Build history of the part. All positions in model axes, mm. Face numbers are marked on the shaded views. A direction names the side the tool comes from. Give positions to 0.01 mm unless a question says otherwise; leave off trailing zeros. Loops run counter-clockwise (first coordinate to the right, second up) from the corner with the lowest first, then second, coordinate; pieces in that order, holes last. Notation, with made-up numbers: (5, 35) -> (17, 35) arc R26 cw to (17, 69) -> close; hole circle Ø5 at (18, 71.5). An arc over 180 degrees is marked (long way). One line per question, with ' | ' between items. Start each with the question number.
(1) 3-axis set-ups, long thin cutter, end or side, ignore diameter. For the marked faces 1, 2 and 3: which of +Z, -Z, +X, -X, +Y, -Y reach the whole face in a straight line?
(2) Slice it at C-C, the plane y = 17. Write the cut outline in (x, z) (3 decimals), then the cut area to 3 significant figures.
(3) Slice it at A-A, the plane z = -3.5. Write the cut outline in (x, y) (3 decimals), then the cut area to 3 significant figures.
(4) Drill centre lines: L1, parallel to Y at x = -22.5, z = 29; L2, parallel to X at y = -26.5, z = -1.5 (3 decimals); L3, parallel to Y at x = 32.5, z = 24.5. Where is each one in solid material? Low to high. Write a range as from..to.
(5) Flat gauge pins, fed straight in: pin 1 Ø2 at (x, y) = (62, 24.5) entering from -Z; pin 2 Ø2 at (x, y) = (60.5, -25) entering from +Z (3 decimals); pin 3 Ø21 at (x, z) = (47.5, 46) entering from -Y; pin 4 Ø24.5 at (x, z) = (-1.5, 40) entering from -Y. Where does each tip first touch, or does it go through?
(6) Slice it at B-B, the plane y = -49.5. Write the cut outline in (x, z) (3 decimals), then the cut area to 3 significant figures.
```python
from build123d import *

# Parameters (mm, degrees)
F1_DEPTH = 63.5
F2_DEPTH = 25.4
F3_DEPTH = 7.9375
F5_R     = 6.35


with BuildPart() as f1:
    # F0 (on Front) → F1 (new body, symmetric)
    with BuildSketch(Plane.XZ):
        Polygon((-41.275, -9.525), (41.275, -9.525), (41.275, 9.525), (22.225, 9.525), (-41.275, 9.525), align=None)
    extrude(amount=F1_DEPTH, both=True)

    # F0 (on Front) → F2 (join, symmetric)
    with BuildSketch(Plane.XZ):
        with BuildLine():
            Line((22.225, 9.525), (41.275, 9.525))
            Line((41.275, 9.525), (41.275, 27.0002))
            ThreePointArc((41.275, 27.0002), (42.449861, 32.993658), (45.800548, 38.1))
            Line((45.800548, 38.1), (42.194617, 38.1))
            Line((42.194617, 38.1), (42.194617, 58.561128))
            ThreePointArc((42.194617, 58.561128), (27.636678, 45.674231), (22.225, 27.0002))
            Line((22.225, 27.0002), (22.225, 9.525))
        make_face()
        with BuildLine():
            ThreePointArc((57.15, 61.9252), (49.485464, 61.073804), (42.194617, 58.561128))
            Line((42.194617, 58.561128), (42.194617, 38.1))
            Line((42.194617, 38.1), (45.800548, 38.1))
            ThreePointArc((45.800548, 38.1), (50.993447, 41.632783), (57.15, 42.8752))
            Line((57.15, 42.8752), (67.442127, 42.8752))
            Line((67.442127, 42.8752), (67.442127, 61.9252))
            Line((67.442127, 61.9252), (57.15, 61.9252))
        make_face()
    extrude(amount=F2_DEPTH, both=True)

    # F0 (on Front) → F3 (join, symmetric)
    with BuildSketch(Plane.XZ):
        with BuildLine():
            add(Edge.make_bspline(
                [(-41.275, 9.525), (-23.330939, 37.566107), (8.143247, 57.774324), (42.194617, 58.561128)],
                knots=[0, 0, 0, 0, 96.807638, 96.807638, 96.807638, 96.807638], degree=3))
            Line((-41.275, 9.525), (22.225, 9.525))
            Line((22.225, 9.525), (22.225, 27.0002))
            ThreePointArc((22.225, 27.0002), (27.636678, 45.674231), (42.194617, 58.561128))
        make_face()
    extrude(amount=F3_DEPTH, both=True)

    # F0 (on Front) → F4 (revolve)
    with BuildSketch(Plane.XZ):
        Polygon((67.442127, 42.8752), (67.442127, 38.1), (92.994617, 38.1), (92.994617, 66.675), (67.442127, 66.675), (67.442127, 61.9252), align=None)
    revolve(axis=Axis((67.442127, 0, 52.3875), (0, 0, -1)))

    # F5
    f5_edges = [f1.edges().sort_by_distance(p)[0] for p in [
        (41.275, -63.5, 0),
        (-41.275, -63.5, 0),
        (41.275, 63.5, 0),
        (-41.275, 63.5, 0),
    ]]
    fillet(f5_edges, radius=F5_R)


solid = f1.part
```
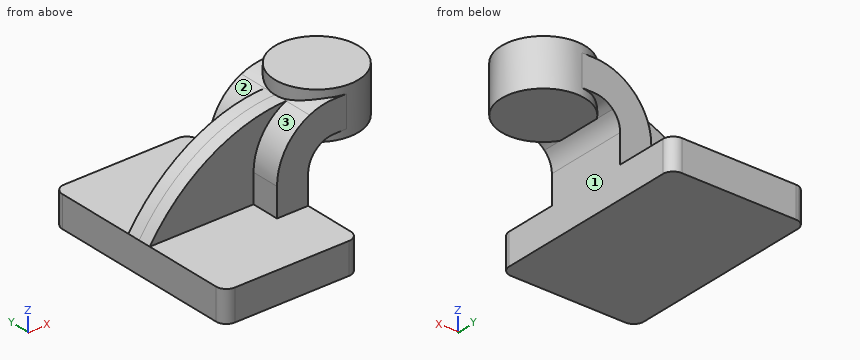
Final values:
1) face 1: -Z, +X, +Y, -Y | face 2: +Z, -X, +Y | face 3: +Z, -X, -Y
2) outline: (-41.275, -9.525) -> (41.275, -9.525) -> (41.275, 27) arc R15.875 cw to (45.801, 38.1) arc R15.875 cw to (48.365, 40.223) -> (48.365, 38.1) -> (86.519, 38.1) -> (86.519, 66.675) -> (48.365, 66.675) -> (48.365, 60.802) arc R34.925 ccw to (42.195, 58.561) arc R34.925 ccw to (22.225, 27) -> (22.225, 9.525) -> (-41.275, 9.525) -> close | area: 3,580 mm2
3) outline: (-41.275, -57.15) arc R6.35 ccw to (-34.925, -63.5) -> (34.925, -63.5) arc R6.35 ccw to (41.275, -57.15) -> (41.275, 57.15) arc R6.35 ccw to (34.925, 63.5) -> (-34.925, 63.5) arc R6.35 ccw to (-41.275, 57.15) -> close | area: 10,400 mm2
4) L1: -7.94..7.94 | L2: -41.275..41.275 | L3: -25.4..25.4
5) pin 1: z = 38.1 | pin 2: z = 66.675 | pin 3: y = -25.4 | pin 4: y = -7.94
6) outline: (-41.275, -9.525) -> (41.275, -9.525) -> (41.275, 9.525) -> (-41.275, 9.525) -> close | area: 1,570 mm2
